Solid Edge part; units mm, degrees
sketch "Sketch1" plane through (0, 0, 0) normal (0, 0, 1) x (1, 0, 0)
  circle A0 centre (0, 0) radius 9.28
extrude "Protrusion1" add sketch "Sketch1" along normal blind 6.63
sketch "Sketch2" plane through (0, 0, 0) normal (0, 0, -1) x (1, 0, 0)
  circle A0 centre (0, 0) radius 5
extrude "Protrusion2" add sketch "Sketch2" along normal blind 12
sketch "Sketch3" plane through (0, 0, -12) normal (0, 0, -1) x (1, 0, 0)
  circle A0 centre (0, 0) radius 4.9997
extrude "Cutout1" cut sketch "Sketch3" against normal blind 11.5 flip side to cut
chamfer "Chamfer_1" distance 0.75 angle 45 1 edges at (-4.9997, 0, -12)
sketch "Sketch4" plane through (0, 0, 6.63) normal (0, 0, 1) x (1, 0, 0)
  line L0 (-4.703, 8) -> (4.703, 8)
extrude "Cutout2" cut sketch "Sketch4" against normal up to next material side at (0, 8.05, 6.63)
pattern_circular "Pattern1" count 6 over 360 about axis through (0, 0, 6.63) along (0, 0, 1) of "Cutout2"
properties part number "213279" material "Stainless Steel, 304"
Here's how the part is built. I have some questions about the finished solid (model axes, mm). A direction names the side the tool comes from. Coordinates: 2 decimals unless noted, no trailing zeros. Order: outer loops, then holes, each group sorted by start corner. A loop starts at its lowest first (then second) coordinate and runs counter-clockwise, first axis right, second up. Notation, with made-up numbers: M 83,44 L 137,44 A9 ccw 137,61 Z; hole C 59,-5 d1. An arc over 180 degrees is marked long. Answer as CSV lines item,"result".
Item 1: For pin 1 (1 mm diameter, centred on y = 1, z = -7, fed in from +X); pin 2 (3 mm diameter, centred on x = 2.5, z = -3, fed in from -Y), each with a flat end and sliding along its axis, tell me the tip position at first contact or that it passes through.
Results found:
pin 1,"x = 4.97"
pin 2,"y = -4.9"
Item 2: If I drill on line 1 (X direction, y = 0, z = -2.5); line 2 (Z direction, x = 4.25, y = 5.5), over which ranges is the centre line in solid material (lowest first)?
Results found:
line 1,"-5 to 5"
line 2,"0 to 6.63"
Item 3: On a 3-axis mill with a long thin cutter (end or side, diameter ignored), from which of +Z, -Z, +X, -X, +Y, -Y can I reach the whole of each face in a straight line? I mean faces 1 (the face through (4, 4, 0)), 2 (the face through (-6.896, 4.056, 3.361)). Say none if no direction works.
Results found:
face 1,"-Z"
face 2,"+Z, -Z, -X, +Y"
Item 4: Imagine slicing it at D-D on z = -10.25. Write out the boundary of the cut face in (x, y).
Results found:
outline,"C 0,0 d10"
Item 5: Imagine slicing it at C-C on y = -5.75. Write out the boundary of the cut face in (x, z).
Results found:
outline,"M -5.92,0 L 5.92,0 L 5.92,6.63 L -5.92,6.63 Z"
Item 6: Imagine slicing it at B-B on z = 1. Write out the boundary of the cut face in (x, y), plus the area to 3 significant figures.
Results found:
outline,"M -9.24,0 L -4.62,-8 L 4.62,-8 L 9.24,0 L 4.62,8 L -4.62,8 Z"
area,"222 mm2"
